Input: part model. Units: mm. Frame: model coordinates. A direction names the side the tool comes from. Give positions to 0.01 mm unless a question says otherwise; leave off trailing zeros. Loops run counter-clockwise (first coordinate to the right, second up) from the corner with the lowest first, then second, coordinate; pieces in that order, holes last. Notation, with made-up numbers: M 49,61 L 55,61 A26 cw 55,91 Z; hole C 14,27.25 d4. An arc over 180 degrees is marked long. Use a Markdown table: item, result. Add a question column.
from build123d import *

# Parameters (mm, degrees)
F0_W     = 38.1
F0_H     = 63.5
F1_DEPTH = 127
F2_W     = 19.05
F2_H     = 12.7
F3_DEPTH = 127.001
F4_W     = 12.7
F4_H     = 25.4
F5_DEPTH = 127.001


with BuildPart() as f1:
    # F0 (on Right) → F1 (new body)
    with BuildSketch(Plane.YZ):
        with Locations((-19.05, 31.75)):
            Rectangle(F0_W, F0_H)
    extrude(amount=F1_DEPTH)

    # F2 (on face) → F3 (cut, through all)
    with BuildSketch(Plane.YZ.offset(127)):
        with Locations((-28.575, 6.35)):
            Rectangle(F2_W, F2_H)
    extrude(amount=-F3_DEPTH, mode=Mode.SUBTRACT)

    # F4 (on face) → F5 (cut, through all)
    with BuildSketch(Plane.YZ.offset(127)):
        with Locations((-19.05, 50.8)):
            Rectangle(F4_W, F4_H)
    extrude(amount=-F5_DEPTH, mode=Mode.SUBTRACT)


solid = f1.part
1) Ray query, line 1 (Y direction, x = 106, z = 50.5); line 2 (Z direction, x = 33.5, y = -30); line 3 (Z direction, x = 92.5, y = -22.5). Return the intervals inside material, ascending. Write a range as [from, to].
2) Section query A-A, the plane z = 53.5. Return the cut outline in (x, y), and give its area (3 significant figures).
3) Section query C-C, the plane y = -23. Return the cut outline in (x, z), and give its area (3 significant figures).
4) Section query B-B, the plane x = 68.5. Return the cut outline in (y, z).
5) Reachability of faces 1 (the flat face through (63, -6, 63.5)), 2 (the flat face through (64, -29, 12.7)), 3 (the flat face through (64, -12.7, 51)) from +Z, -Z, +X, -X, +Y, -Y: full face, straight path, thin tool, end or side. Return the list, or none.
6) Pull-direction query (Y, two-part tool) for faces 4 (the flat face through (64, -25.4, 51)), 5 (the flat face through (64, -19.05, 6)), 6 (the flat face through (127, -19, 32)); classes: pulls with the +Y half, pulls with the -Y half, needs draft (parallel to the pull), parting line crosses it, or undercut.
7) Section query D-D, the plane z = 9.5. Return the cut outline in (x, y).
8) Contact query for flat-ended pins moving along their axis: P1, Ø10, axis at x = 57.5, z = 5, coming from the -Y side; P2, Ø9.5, axis at x = 51.5, y = -26.5, coming from the -Z side; P3, Ø2, axis at x = 90, y = -23, coming from the +Z side. Output: stop coordinate, or through.
Entries:
| question | item | result |
|---|---|---|
| 1 | line 1 | y = [-38.1, -25.4], [-12.7, 0] |
| 1 | line 2 | z = [12.7, 63.5] |
| 1 | line 3 | z = [12.7, 38.1] |
| 2 | outline | M 0,-38.1 L 127,-38.1 L 127,-25.4 L 0,-25.4 Z; M 0,-12.7 L 127,-12.7 L 127,0 L 0,0 Z |
| 2 | area | 3,230 mm² |
| 3 | outline | M 0,12.7 L 127,12.7 L 127,38.1 L 0,38.1 Z |
| 3 | area | 3,230 mm² |
| 4 | outline | M -38.1,12.7 L -19.05,12.7 L -19.05,0 L 0,0 L 0,63.5 L -12.7,63.5 L -12.7,38.1 L -25.4,38.1 L -25.4,63.5 L -38.1,63.5 Z |
| 5 | face 1 | +Z, +X, -X, +Y, -Y |
| 5 | face 2 | -Z, +X, -X, -Y |
| 5 | face 3 | +Z, +X, -X |
| 6 | face 4 | undercut |
| 6 | face 5 | pulls with the -Y half |
| 6 | face 6 | needs draft |
| 7 | outline | M 0,-19.05 L 127,-19.05 L 127,0 L 0,0 Z |
| 8 | P1 | stops at y = -19.05 |
| 8 | P2 | stops at z = 12.7 |
| 8 | P3 | stops at z = 38.1 |
